Source: CAD feature listing. Evaluate the final solid. Frame: model axes, mm. A direction names the side the tool comes from. Coordinates: 2 decimals unless noted, no trailing zeros. Order: outer loops, then holes, each group sorted by start corner. A loop starts at its lowest first (then second) coordinate and runs counter-clockwise, first axis right, second up. Notation, with made-up numbers: (-20.75, -35) - (3.25, -35) arc R29 cw to (3.25, -8) - close; hole circle Ø8 at (80.25, -31.5). An arc over 180 degrees is marked (long way). One line per question, with ' | ' between items.
Autodesk Inventor part; units mm, degrees
ref_plane "YZ Plane" through (0, 0, 0) normal (1, 0, 0) x (0, 1, 0)
ref_plane "XZ Plane" through (0, 0, 0) normal (0, 1, 0) x (-1, 0, 0)
ref_plane "XY Plane" through (0, 0, 0) normal (0, 0, 1) x (1, 0, 0)
sketch "草圖1" plane through (0, 0, 0) normal (0, 1, 0) x (-1, 0, 0)
  line L0 (2.5, 2.5) -> (-2.5, 2.5)
  line L1 (-2.5, 2.5) -> (-2.5, -2.5)
  line L2 (-2.5, -2.5) -> (2.5, -2.5)
  line L3 (2.5, -2.5) -> (2.5, 2.5)
  circle A0 centre (0, 0) radius 1.7
  point P0 (0, -2.5)
  point P1 (2.5, 0)
  dimension "d0" = 5
  dimension "d1" = 5
  dimension "d2" = 3.4
sketch "草圖2" plane through (0, 0, 0) normal (1, 0, 0) x (0, 1, 0)
  line L0 (0, -2.5) -> (0, 2.5)
  line L1 (5, -2.5) -> (0, -2.5)
  line L2 (0, 0) -> (1.5, 0)
  line L3 (0, 2.5) -> (2, 2.5)
  line L4 (2, 2.5) -> (5, -2.5)
  point P0 (0, 2.5)
  dimension "d3" = 1.5
  dimension "d7" = 2
  dimension "d8" = 5
extrude "擠出1" add sketch "草圖2" along normal mid plane 5
extrude "擠出2" cut sketch "草圖1" along normal blind 1.5 contours A0
properties part number "110033226_ipt_14_草地三"
(1) Cut plane C-C (x = 0). Return the cut outline in (y, z), and give its area (3 significant figures).
Taken from the geometry:
outline: (0, -2.5) - (5, -2.5) - (2, 2.5) - (0, 2.5) - (0, 1.7) - (1.5, 1.7) - (1.5, -1.7) - (0, -1.7) - close | area: 12.4 mm²
(2) Cut plane B-B (y = 0.6). Return the cut outline in (x, z), and give its area (3 significant figures).
Taken from the geometry:
outline: (-2.5, -2.5) - (2.5, -2.5) - (2.5, 2.5) - (-2.5, 2.5) - close; hole circle Ø3.4 at (0, 0) | area: 15.9 mm²
(3) Pull-direction query (Z, two-part tool) for faces 3 (the cylindrical face through (0.37, 0.74, 1.66)), 4 (the flat face through (0, 3, -2.5)), 5 (the flat face through (0, 1, 2.5)); classes: pulls with the +Z half, pulls with the -Z half, needs draft (parallel to the pull), parting line crosses it, or undercut.
Taken from the geometry:
face 3: undercut | face 4: pulls with the -Z half | face 5: pulls with the +Z half
(4) Cut plane A-A (z = 0). Return the cut outline in (x, y), and give its area (3 significant figures).
Taken from the geometry:
outline: (-2.5, 0) - (-1.7, 0) - (-1.7, 1.5) - (1.7, 1.5) - (1.7, 0) - (2.5, 0) - (2.5, 3.5) - (-2.5, 3.5) - close | area: 12.4 mm²
(5) Set-up query: faces 1 (the flat face through (0, 3.5, 0)), 2 (the flat face through (0, 1.5, 0)). Return all of +Z, -Z, +X, -X, +Y, -Y with unobstructed straight access to the full face (end or side cutting, diameter ignored); none if empty.
Taken from the geometry:
face 1: +Z, +X, -X, +Y | face 2: -Y
(6) Cut plane D-D (y = 3.35). Return the cut outline in (x, z).
Taken from the geometry:
outline: (-2.5, -2.5) - (2.5, -2.5) - (2.5, 0.25) - (-2.5, 0.25) - close
(7) Material intervals for L1, parallel to Z at x = 0, y = 1.2; L2, parallel to Z at x = -1.8, y = 2.3; L3, parallel to Z at x = 1.35, y = 1.45, sorted ascending. Write a range as from..to.
Taken from the geometry:
L1: z = -2.5..-1.7, 1.7..2.5 | L2: z = -2.5..2 | L3: z = -2.5..-1.03, 1.03..2.5
